Model file for the job. Use its own axes, mm. A direction names the side the tool comes from. Coordinates: 2 decimals unless noted, no trailing zeros. Order: outer loops, then holes, each group sorted by start corner. A loop starts at its lowest first (then second) coordinate and runs counter-clockwise, first axis right, second up. Notation, with made-up numbers: (38, 87.5) -> (52, 87.5) arc R18 ccw to (52, 115.5) -> close; hole circle Ø1 at (7, 76.5). An arc over 180 degrees is marked (long way). Use CSV: the item, a comma, the result in double quotes. Start each with the question number.
(1) Cut at A-A on x = 0. Write the cut outline in (y, z) (1 decimal), plus the area to 3 significant figures.
(2) Cut at C-C on z = 0. Write the cut outline in (x, y) (1 decimal), plus the area to 3 significant figures.
(3) Cut at B-B on y = 9.5. Write the cut outline in (x, z) (3 decimals), plus the area to 3 significant figures.
(4) Cut at D-D on x = 25. Write the cut outline in (y, z).
(5) Pin check, flat tips, straight feed: pin 1 Ø1.5 at (y, z) = (1.5, -7.5) entering from +X; pin 2 Ø3 at (x, y) = (-18.5, -0.5) entering from -Z; pin 3 Ø11 at (x, z) = (10.07, -17.45) entering from +Y; pin 4 Ø11 at (x, z) = (10.07, 17.45) entering from -Y. Stop position of each tip, or through.
(6) Tool access for faces 4 (the flat face through (-17.063, 5.691, 4.976)), 5 (the flat face through (17.063, 5.691, 4.976)), 6 (the cylindrical face through (-12.844, -3.046, 15.321)), 7 (the flat face through (-12.84, 5.69, -12.29)), 8 (the flat face through (-7, 0, 13)): list every direction of +Z, -Z, +X, -X, +Y, -Y with a clear straight run to the whole face (end or side of a thin tool).
(7) Pull direction Z, two halves, no side cores. Call faces 1 (the flat face through (-10, 0, -4)), 2 (the flat face through (-13, -6.007, 0)), 3 (the conical face through (-0.089, 9.003, -18.011)): pulls with the +Z half, pulls with the -Z half, needs draft (parallel to the pull), parting line crosses it, or undercut.
(8) Probe L1, parallel to X at y = -2, z = 0; L2, parallel to X at y = 7, z = 0 (3 decimals); L3, parallel to Z at x = 0, y = -2.5. List the from-to ranges inside material, lowest first.
Autodesk Inventor part; units mm, degrees
ref_plane "YZ Plane" through (0, 0, 0) normal (1, 0, 0) x (0, 1, 0)
ref_plane "XZ Plane" through (0, 0, 0) normal (0, 1, 0) x (-1, 0, 0)
ref_plane "XY Plane" through (0, 0, 0) normal (0, 0, 1) x (1, 0, 0)
sketch "Sketch1" plane through (0, 0, 0) normal (0, 0, 1) x (1, 0, 0)
  line L0 (0, 52.767) -> (0, -45.7542)
  line L1 (-13.335, 25.4) -> (-13.335, 0)
  line L2 (-10.5093, 0) -> (-10.5092, -6.0071)
  line L3 (-13.335, 0) -> (-10.5093, 0)
  line L4 (-13.335, 25.4) -> (-14.605, 25.4)
  line L5 (-14.605, 25.4) -> (-14.605, 14.903)
  line L6 (-10.5092, -6.0071) -> (-29.7815, -6.0071)
  line L7 (-29.7815, -6.0071) -> (-29.7815, 0)
  line L8 (-29.7815, 0) -> (-23.2093, 0)
  line L9 (-23.2093, 0) -> (-14.605, 14.903)
  point P0 (0, 0)
  dimension "d0" = 25.4
  dimension "d1" = 26.67
  dimension "d2" = 6.0071
  dimension "d3" = 21.0185
  dimension "d4" = 1.27
  dimension "d5" = 19.2722
  dimension "d6" = 6.5723
  dimension "d7" = 30
revolve "Revolution1" add sketch "Sketch1" angle 360 about axis through (0, 52.767, 0) along (0, -1, 0)
sketch "Sketch2" plane through (0, -6.0071, 0) normal (0, -1, 0) x (1, 0, 0)
  circle A0 centre (0, 0) radius 10.5093
  circle A1 centre (0, 0) radius 10.5092
  circle A2 centre (0, 0) radius 29.7815
  circle A3 centre (0, 0) radius 20.1454
  circle A4 centre (0, 0) radius 29.7815
  line L0 (29.7815, 0) -> (20.1454, 0)
  line L1 (-10.5093, 0) -> (-20.1454, 0)
  circle A5 centre (20.1454, 0) radius 3.4925
  circle A6 centre (10.0727, 17.4464) radius 3.4925
  circle A7 centre (-10.0727, 17.4464) radius 3.4925
  circle A8 centre (-20.1454, 0) radius 3.4925
  circle A9 centre (-10.0727, -17.4464) radius 3.4925
  circle A10 centre (10.0727, -17.4464) radius 3.4925
  point P0 (0, 0)
  dimension "d10" = 6.985
  dimension "d13" = 360
extrude "Extrusion1" cut sketch "Sketch2" against normal through all contours A8 A3 L1 | L1 A3 A8 | A3 A8 | A7 A3 | A3 A7 | A9 A3 | A3 A9 | A6 A3 | A3 A6 | A10 A3 | A3 A10 | A5 L0 A3 | A3 A5 | A3 L0 A5
sketch "Sketch3" plane through (0, 0, 0) normal (0, 1, 0) x (1, 0, 0)
  circle A0 centre (0, 0) radius 29.7815
  arc A1 (26.4165, -13.7516) -> (26.4165, 13.7516) centre (0, 0) ccw
  line L0 (14.3942, 2.4722) -> (26.4165, 13.7516)
  line L1 (14.3942, -2.4722) -> (26.4165, -13.7516)
  circle A2 centre (0, 0) radius 14.605
  arc A3 (14.3942, -2.4722) -> (14.3942, 2.4722) centre (0, 0) ccw
  arc A4 (25.1175, 16.0016) -> (1.2991, 29.7532) centre (0, 0) ccw
  line L2 (5.0561, 13.7019) -> (1.2991, 29.7532)
  line L3 (9.3381, 11.2297) -> (25.1175, 16.0016)
  arc A5 (9.3381, 11.2297) -> (5.0561, 13.7019) centre (0, 0) ccw
  arc A6 (-1.2991, 29.7532) -> (-25.1175, 16.0016) centre (0, 0) ccw
  line L4 (-9.3381, 11.2297) -> (-25.1175, 16.0016)
  line L5 (-5.0561, 13.7019) -> (-1.2991, 29.7532)
  arc A7 (-5.0561, 13.7019) -> (-9.3381, 11.2297) centre (0, 0) ccw
  arc A8 (-26.4165, 13.7516) -> (-26.4165, -13.7516) centre (0, 0) ccw
  line L6 (-14.3942, -2.4722) -> (-26.4165, -13.7516)
  line L7 (-14.3942, 2.4722) -> (-26.4165, 13.7516)
  arc A9 (-14.3942, 2.4722) -> (-14.3942, -2.4722) centre (0, 0) ccw
  arc A10 (-25.1175, -16.0016) -> (-1.2991, -29.7532) centre (0, 0) ccw
  line L8 (-5.0561, -13.7019) -> (-1.2991, -29.7532)
  line L9 (-9.3381, -11.2297) -> (-25.1175, -16.0016)
  arc A11 (-9.3381, -11.2297) -> (-5.0561, -13.7019) centre (0, 0) ccw
  arc A12 (1.2991, -29.7532) -> (25.1175, -16.0016) centre (0, 0) ccw
  line L10 (9.3381, -11.2297) -> (25.1175, -16.0016)
  line L11 (5.0561, -13.7019) -> (1.2991, -29.7532)
  arc A13 (5.0561, -13.7019) -> (9.3381, -11.2297) centre (0, 0) ccw
  line L12 (-2.8655, 0) -> (7.3025, 0)
  point P0 (23.1395, -1.798)
  point P1 (23.1395, 1.798)
  point P2 (19.5399, 3.4396)
  point P3 (19.5399, -3.4396)
  point P4 (13.1269, 19.1404)
  point P5 (10.0126, 20.9384)
  point P6 (-10.0126, 20.9384)
  point P7 (-13.1269, 19.1404)
  point P8 (-23.1395, 1.798)
  point P9 (-23.1395, -1.798)
  point P10 (-13.1269, -19.1404)
  point P11 (-10.0126, -20.9384)
  point P12 (10.0126, -20.9384)
  point P13 (13.1269, -19.1404)
  point P14 (-5.0561, 13.7019)
  point P15 (-1.2991, 29.7532)
  point P16 (-25.1175, 16.0016)
  point P17 (-9.3381, 11.2297)
  point P18 (-14.3942, 2.4722)
  point P19 (-26.4165, 13.7516)
  point P20 (-26.4165, -13.7516)
  point P21 (-14.3942, -2.4722)
  point P22 (-9.3381, -11.2297)
  point P23 (-25.1175, -16.0016)
  point P24 (-1.2991, -29.7532)
  point P25 (-5.0561, -13.7019)
  point P26 (5.0561, -13.7019)
  point P27 (1.2991, -29.7532)
  point P28 (25.1175, -16.0016)
  point P29 (9.3381, -11.2297)
  point P30 (9.3381, 11.2297)
  point P31 (1.2991, 29.7532)
  point P32 (5.0561, 13.7019)
  dimension "d21" = 360
  dimension "d23" = 55
extrude "Extrusion2" cut sketch "Sketch3" along normal blind 25.4 contours A0 L1 A2 L0 | L3 A2 L2 A0 | A0 L11 A2 L10 | L5 A2 L4 A0 | A0 L9 A2 L8 | L7 A2 L6 A0
properties part number "Connector_ring"
Outcome:
1,outline,"(-6, -29.8) -> (0, -29.8) -> (0, -23.2) -> (14.9, -14.6) -> (25.4, -14.6) -> (25.4, -13.3) -> (0, -13.3) -> (0, -10.5) -> (-6, -10.5) -> close; (-6, 10.5) -> (0, 10.5) -> (0, 13.3) -> (25.4, 13.3) -> (25.4, 14.6) -> (14.9, 14.6) -> (0, 23.2) -> (0, 29.8) -> (-6, 29.8) -> close"
1,area,"424 mm2"
2,outline,"(-29.8, -6) -> (-23.6, -6) -> (-23.6, 0) -> (-29.8, 0) -> close; (-16.7, -6) -> (-10.5, -6) -> (-10.5, 0) -> (-13.3, 0) -> (-13.3, 25.4) -> (-14.6, 25.4) -> (-14.6, 0) -> (-16.7, 0) -> close; (10.5, -6) -> (16.7, -6) -> (16.7, 0) -> (14.6, 0) -> (14.6, 25.4) -> (13.3, 25.4) -> (13.3, 0) -> (10.5, 0) -> close; (23.6, -6) -> (29.8, -6) -> (29.8, 0) -> (23.6, 0) -> close"
2,area,"212 mm2"
3,outline,"(-17.023, -4.938) arc R17.724 ccw to (-12.788, -12.273) -> (-9.338, -11.23) arc R14.605 ccw to (-5.056, -13.702) -> (-4.235, -17.211) arc R17.724 ccw to (4.235, -17.211) -> (5.056, -13.702) arc R14.605 ccw to (9.338, -11.23) -> (12.788, -12.273) arc R17.724 ccw to (17.023, -4.938) -> (14.394, -2.472) arc R14.605 ccw to (14.394, 2.472) -> (17.023, 4.938) arc R17.724 ccw to (12.788, 12.273) -> (9.338, 11.23) arc R14.605 ccw to (5.056, 13.702) -> (4.235, 17.211) arc R17.724 ccw to (-4.235, 17.211) -> (-5.056, 13.702) arc R14.605 ccw to (-9.338, 11.23) -> (-12.788, 12.273) arc R17.724 ccw to (-17.023, 4.938) -> (-14.394, 2.472) arc R14.605 ccw to (-14.394, -2.472) -> close; hole circle Ø26.67 at (0, 0)"
3,area,"288 mm2"
4,outline,"(-6.01, -16.18) -> (0, -16.18) -> (0, 16.18) -> (-6.01, 16.18) -> close"
5,pin 1,"x = 20.55"
5,pin 2,"z = -24.45"
5,pin 3,"y = 0"
5,pin 4,"y = -6.01"
6,face 4,"-X, +Y"
6,face 5,"+X, +Y"
6,face 6,"+Y, -Y"
6,face 7,"-Z, +Y"
6,face 8,"+Y"
7,face 1,"undercut"
7,face 2,"needs draft"
7,face 3,"pulls with the -Z half"
8,L1,"-29.78 to -23.64, -16.65 to -10.51, 10.51 to 16.65, 23.64 to 29.78"
8,L2,"-14.605 to -13.335, 13.335 to 14.605"
8,L3,"-29.78 to -10.51, 10.51 to 29.78"
